from build123d import *

# Parameters (mm, degrees)
F0_R      = 6.5
F1_DEPTH  = 3
F2_DEPTH  = 10
F4_D      = 3.3
F4_DEPTH  = 8
F4_TIP    = 0.9914200214
F5_D      = 5.8
F5_DEPTH  = 1.5
F5_TIP    = 1.7424957952
F6_START  = -4
F6_DEPTH  = 2
F8_START  = -4
F8_DEPTH  = 2
F9_D      = 5.8
F9_DEPTH  = 1.5
F9_TIP    = 1.7424957952
F10_D     = 3.3
F10_DEPTH = 8
F10_START = 2.2510758
F10_TIP   = 0.9914200214
F12_START = -4
F12_DEPTH = 2
F13_D     = 3.3
F13_DEPTH = 8
F13_TIP   = 0.9914200214
F14_D     = 5.8
F14_DEPTH = 1.5
F14_TIP   = 1.7424957952
F15_R     = 2
F16_DEPTH = 8
F17_D     = 5.1054
F17_DEPTH = 15.81
F17_TIP   = 1.5338169022


with BuildPart() as f1:
    # F0 (on Front) → F1 (new body)
    with BuildSketch(Plane.XZ):
        Polygon((-0.0364092433, -16.1657665361), (14.0181691136, 8.0513519384), (-13.9817598703, 8.1144145977), align=None)
        Circle(F0_R, mode=Mode.SUBTRACT)
    extrude(amount=F1_DEPTH)

    # F0 (on Front) → F2 (join)
    with BuildSketch(Plane.XZ):
        Polygon((-0.0595551194, -26.4425752627), (22.9297194786, 13.169711385), (-22.8701643592, 13.2728638777), align=None)
        Polygon((-13.9817598703, 8.1144145977), (14.0181691136, 8.0513519384), (-0.0364092433, -16.1657665361), align=None, mode=Mode.SUBTRACT)
    extrude(amount=F2_DEPTH)

    # F4
    with Locations(Plane(origin=(11.4350821796, 0, -6.6364319388), x_dir=(0, 1, 0), z_dir=(0.8648970884, 0, -0.501949227))):
        with Locations((-5, -8.5), (-5, 8.5)):
            Hole(F4_D / 2, depth=F4_DEPTH)
            with Locations((0, 0, -(F4_DEPTH + F4_TIP / 2))):  # 118° drill point
                Cone(0, F4_D / 2, F4_TIP, mode=Mode.SUBTRACT)

    # F5
    with Locations(Plane(origin=(11.4350821796, 0, -6.6364319388), x_dir=(0, 1, 0), z_dir=(0.8648970884, 0, -0.501949227))):
        with Locations((-5, -8.5), (-5, 8.5)):
            Hole(F5_D / 2, depth=F5_DEPTH)
            with Locations((0, 0, -(F5_DEPTH + F5_TIP / 2))):  # 118° drill point
                Cone(0, F5_D / 2, F5_TIP, mode=Mode.SUBTRACT)

    # F3 (on face) → F6 (cut)
    with BuildSketch(Plane(origin=(11.4350821796, 0, -6.6364319388), x_dir=(0, 1, 0), z_dir=(0.8648970884, 0, -0.501949227)).offset(F6_START)):
        Polygon((-2.1, -10.1743157806), (-2.1, -6.8256842194), (-5, -5.1513684387), (-7.9, -6.8256842194), (-7.9, -10.1743157806), (-5, -11.8486315613), align=None)
        Polygon((-2.1, 6.8256842194), (-2.1, 10.1743157806), (-5, 11.8486315613), (-7.9, 10.1743157806), (-7.9, 6.8256842194), (-5, 5.1513684387), align=None)
    extrude(amount=-F6_DEPTH, mode=Mode.SUBTRACT)

    # F7 (on face) → F8 (cut)
    with BuildSketch(Plane(origin=(0.0297775597, 0, 13.2212876313), x_dir=(0.9999974637, 0, -0.0022522378), z_dir=(0.0022522378, 0, 0.9999974637)).offset(F8_START)):
        Polygon((6.8256842194, -2.1), (5.1513684387, -5), (6.8256842194, -7.9), (10.1743157806, -7.9), (11.8486315613, -5), (10.1743157806, -2.1), align=None)
        Polygon((-10.1743157806, -2.1), (-11.8486315613, -5), (-10.1743157806, -7.9), (-6.8256842194, -7.9), (-5.1513684387, -5), (-6.8256842194, -2.1), align=None)
    extrude(amount=-F8_DEPTH, mode=Mode.SUBTRACT)

    # F9
    with Locations(Plane(origin=(0.0297775597, 0, 13.2212876313), x_dir=(0.9999974637, 0, -0.0022522378), z_dir=(0.0022522378, 0, 0.9999974637))):
        with Locations((8.5, -5), (-8.5, -5)):
            Hole(F9_D / 2, depth=F9_DEPTH)
            with Locations((0, 0, -(F9_DEPTH + F9_TIP / 2))):  # 118° drill point
                Cone(0, F9_D / 2, F9_TIP, mode=Mode.SUBTRACT)

    # F10
    # its depths count from where the whole tool has entered the part; down to there all is cleared
    with Locations(Plane(origin=(0.0297775597, 0, 13.2212876313), x_dir=(0.9999974637, 0, -0.0022522378), z_dir=(0.0022522378, 0, 0.9999974637)).offset(-F10_START)):
        with Locations((8.5, -5), (-8.5, -5)):
            Hole(F10_D / 2, depth=F10_DEPTH)
            with Locations((0, 0, -(F10_DEPTH + F10_TIP / 2))):  # 118° drill point
                Cone(0, F10_D / 2, F10_TIP, mode=Mode.SUBTRACT)

    # F11 (on face) → F12 (cut)
    with BuildSketch(Plane(origin=(-11.4648597393, 0, -6.5848556925), x_dir=(0, -1, 0), z_dir=(-0.8671493262, 0, -0.4980482367)).offset(F12_START)):
        Polygon((2.1, 6.8256842194), (5, 5.1513684387), (7.9, 6.8256842194), (7.9, 10.1743157806), (5, 11.8486315613), (2.1, 10.1743157806), align=None)
        Polygon((2.1, -10.1743157806), (5, -11.8486315613), (7.9, -10.1743157806), (7.9, -6.8256842194), (5, -5.1513684387), (2.1, -6.8256842194), align=None)
    extrude(amount=-F12_DEPTH, mode=Mode.SUBTRACT)

    # F13
    with Locations(Plane(origin=(-11.4648597393, 0, -6.5848556925), x_dir=(0, -1, 0), z_dir=(-0.8671493262, 0, -0.4980482367))):
        with Locations((5, 8.5), (5, -8.5)):
            Hole(F13_D / 2, depth=F13_DEPTH)
            with Locations((0, 0, -(F13_DEPTH + F13_TIP / 2))):  # 118° drill point
                Cone(0, F13_D / 2, F13_TIP, mode=Mode.SUBTRACT)

    # F14
    with Locations(Plane(origin=(-11.4648597393, 0, -6.5848556925), x_dir=(0, -1, 0), z_dir=(-0.8671493262, 0, -0.4980482367))):
        with Locations((5, 8.5), (5, -8.5)):
            Hole(F14_D / 2, depth=F14_DEPTH)
            with Locations((0, 0, -(F14_DEPTH + F14_TIP / 2))):  # 118° drill point
                Cone(0, F14_D / 2, F14_TIP, mode=Mode.SUBTRACT)

    # F15
    f15_edges = [f1.edges().sort_by_distance(p)[0] for p in [
        (-22.870164, -5, 13.272864),
        (-0.059555, -5, -26.442575),
        (22.929719, -5, 13.169711),
    ]]
    fillet(f15_edges, radius=F15_R)

    # F0 (on Front) → F16 (join)
    with BuildSketch(Plane.XZ):
        Circle(F0_R)
    extrude(amount=F16_DEPTH)

    # F17
    with Locations(Plane(origin=(0, 0, 0), x_dir=(1, 0, 0), z_dir=(0, 1, 0))):
        with Locations((0, 0)):
            Hole(F17_D / 2, depth=F17_DEPTH)
            with Locations((0, 0, -(F17_DEPTH + F17_TIP / 2))):  # 118° drill point
                Cone(0, F17_D / 2, F17_TIP, mode=Mode.SUBTRACT)


solid = f1.part
Model file for the job. Use its own axes, mm. A direction names the side the tool comes from. Give positions to 0.01 mm unless a question says otherwise; leave off trailing zeros. Write each loop counter-clockwise with the first axis right and the second up, starting at its lowest first coordinate (ties: lowest second). Pieces come first, ordered by that corner, then holes. Notation, with made-up numbers: (42, 53.25) - (64, 53.25) arc R22 cw to (64, 81.25) - close; hole circle Ø5 at (-29, -32.5). An arc over 180 degrees is marked (long way). Answer as CSV lines item,"result".
1. Band-saw the part on C-C (z = -6). Write the cut outline in (x, y), and give its area (3 significant figures).
Responses:
outline,"(-11.8, -10) - (-5.88, -10) - (-5.88, -3) - (-2.5, -3) - (-2.5, -8) - (2.5, -8) - (2.5, -3) - (5.86, -3) - (5.86, -10) - (11.8, -10) - (11.8, 0) - (-11.8, 0) - close"
area,"179 mm2"
2. Band-saw the part on D-D (z = -18.5). Write the cut outline in (x, y), and give its area (3 significant figures).
Responses:
outline,"(-4.62, -10) - (4.55, -10) - (4.55, 0) - (-4.62, 0) - close"
area,"91.7 mm2"
3. Pin check, flat tips, straight feed: pin 1 (7.5 mm diameter, centred on x = 2, z = -3, fed in from -Y); pin 2 (3 mm diameter, centred on y = -3, z = -18, fed in from +X); pin 3 (6 mm diameter, centred on x = 9.5, y = -3.5, fed in from +Z). Stop position of each tip, or through.
Responses:
pin 1,"stops at y = -8"
pin 2,"stops at x = 5.71"
pin 3,"stops at z = 13.21"
4. Band-saw the part on A-A (y = -8.5). Write the cut outline in (x, z).
Responses:
outline,"(-21.14, 10.27) - (-1.78, -23.44) arc R2 ccw to (1.68, -23.45) - (21.19, 10.17) arc R2 ccw to (19.47, 13.18) - (-19.41, 13.27) arc R2 ccw to start; hole (-13.98, 8.11) - (-0.04, -16.17) - (14.02, 8.05) - close"
5. Drill centre lines: L1, parallel to Z at x = 2, y = -6; L2, parallel to X at y = -4.5, z = 10; L3, parallel to Y at x = -3, z = -13. Where is each one in solid material? Low to high. Write a range as [from, to].
Responses:
L1,"z = [-22.89, -14.19], [-6.18, -1.59], [1.59, 6.18], [8.08, 13.22]"
L2,"x = [-20.99, -10.05], [-6.91, 6.95], [10.09, 21.09]"
L3,"y = [-10, -7.9], [-2.1, 0]"
6. Band-saw the part on B-B (y = -4.5). Count the separate pieces of the cut face and the enclosed holes in it, and give its area (3 significant figures).
Responses:
separate pieces,"7"
enclosed holes,"1"
area,"527 mm2"
7. 3-axis set-ups, long thin cutter, end or side, ignore diameter. For faces 1 (the face through (-2.435, -4.056, -0.767)), 2 (the face through (-3, -2.1, -11)): which of +Z, -Z, +X, -X, +Y, -Y reach the whole face in a straight line?
Responses:
face 1,"+Y, -Y"
face 2,"none"
8. Two-plate mould, pull along Y, no slides. Class faces 3 (the face through (4.49, -3.35, -12.35)), 4 (the face through (7.09, -7.23, -3.89)): +Y half, -Y half, draft (parallel to the pull), parting line (faces both ways), or undercut.
Responses:
face 3,"undercut"
face 4,"draft"
